For this review, take the finished solid that the model builds, in its own axes (mm). Coordinates: 2 decimals unless noted, no trailing zeros. Write each loop counter-clockwise with the first axis right and the second up, starting at its lowest first coordinate (ties: lowest second). Pieces come first, ordered by that corner, then holes. Notation, with made-up numbers: M 88,46 L 98,46 A16 cw 98,66 Z; hole C 33.5,72 d9. An arc over 180 degrees is marked long. One line per question, with ' | ' between items.
from build123d import *

# Parameters (mm, degrees)
F0_R     = 10.95
F1_DEPTH = 7
F2_R     = 1


with BuildPart() as f1:
    # F0 (on Top) → F1 (new body)
    with BuildSketch(Plane.XY):
        with BuildLine():
            ThreePointArc((-21.5356414958, -4.8959657474), (-23.8783924252, 3.2977389637), (-21.5356414958, 11.4914436749))
            ThreePointArc((-21.5356414958, 11.4914436749), (-22.6993144087, 13.1854483171), (-24.0705316121, 14.7163140059))
            ThreePointArc((-24.0705316121, 14.7163140059), (-24.150511625, 14.7916467191), (-24.2283924252, 14.8691476939))
            ThreePointArc((-24.2283924252, 14.8691476939), (-29.3261886183, 18.1493809552), (-35.2783924252, 19.2977389637))
            ThreePointArc((-35.2783924252, 19.2977389637), (-37.8102942344, 19.0961399344), (-40.2783924252, 18.4964231173))
            ThreePointArc((-40.2783924252, 18.4964231173), (-50.1108366069, -2.7021443349), (-28.305201053, -11.1027680443))
            ThreePointArc((-28.305201053, -11.1027680443), (-26.1407697818, -9.8363332314), (-24.200803492, -8.2472609682))
            ThreePointArc((-24.200803492, -8.2472609682), (-24.1495735944, -8.1967605248), (-24.0974438172, -8.14718953))
            ThreePointArc((-24.0974438172, -8.14718953), (-22.7109617539, -6.6047701285), (-21.5356414958, -4.8959657474))
        make_face()
        with Locations((-35.2783924252, 3.2977389637)):
            Circle(F0_R, mode=Mode.SUBTRACT)
        with BuildLine():
            ThreePointArc((-35.2783924252, 19.2977389637), (-13.6974768248, 21.3714318141), (6.7324567843, 14.1151288356))
            ThreePointArc((6.7324567843, 14.1151288356), (8.5674737327, 15.8243194809), (10.647013196, 17.2257956612))
            ThreePointArc((10.647013196, 17.2257956612), (-14.6417402019, 24.8328180176), (-40.2783924252, 18.4964231173))
            ThreePointArc((-40.2783924252, 18.4964231173), (-37.8102942344, 19.0961399344), (-35.2783924252, 19.2977389637))
        make_face()
        with BuildLine():
            ThreePointArc((-19.2986991166, 4.1035936434), (-8.3783924252, 14.2477389637), (2.5419142663, 4.1035936434))
            ThreePointArc((2.5419142663, 4.1035936434), (3.2081819329, 7.93443985), (4.7788566455, 11.4914436749))
            ThreePointArc((4.7788566455, 11.4914436749), (3.7989548826, 12.8874320009), (2.6716075748, 14.1673065724))
            ThreePointArc((2.6716075748, 14.1673065724), (-8.3783924252, 18.7977389637), (-19.4283924252, 14.1673065724))
            ThreePointArc((-19.4283924252, 14.1673065724), (-20.5557397329, 12.8874320009), (-21.5356414958, 11.4914436749))
            ThreePointArc((-21.5356414958, 11.4914436749), (-19.9649667832, 7.93443985), (-19.2986991166, 4.1035936434))
        make_face()
        with BuildLine():
            ThreePointArc((-19.2986991166, 2.4918842841), (-19.3283924252, 3.2977389637), (-19.2986991166, 4.1035936434))
            ThreePointArc((-19.2986991166, 4.1035936434), (-19.9649667832, 7.93443985), (-21.5356414958, 11.4914436749))
            ThreePointArc((-21.5356414958, 11.4914436749), (-23.8783924252, 3.2977389637), (-21.5356414958, -4.8959657474))
            ThreePointArc((-21.5356414958, -4.8959657474), (-19.9649667832, -1.3389619226), (-19.2986991166, 2.4918842841))
        make_face()
        with BuildLine():
            ThreePointArc((4.7788566455, -4.8959657474), (3.2081819329, -1.3389619226), (2.5419142663, 2.4918842841))
            ThreePointArc((2.5419142663, 2.4918842841), (-8.3783924252, -7.6522610363), (-19.2986991166, 2.4918842841))
            ThreePointArc((-19.2986991166, 2.4918842841), (-19.9649667832, -1.3389619226), (-21.5356414958, -4.8959657474))
            ThreePointArc((-21.5356414958, -4.8959657474), (-20.5557397329, -6.2919540734), (-19.4283924252, -7.571828645))
            ThreePointArc((-19.4283924252, -7.571828645), (-8.3783924252, -12.2022610363), (2.6716075748, -7.571828645))
            ThreePointArc((2.6716075748, -7.571828645), (3.7989548826, -6.2919540734), (4.7788566455, -4.8959657474))
        make_face()
        with BuildLine():
            ThreePointArc((2.5419142663, 4.1035936434), (2.5641817297, 3.7009397379), (2.5716075748, 3.2977389637))
            ThreePointArc((2.5716075748, 3.2977389637), (2.5641817297, 2.8945381895), (2.5419142663, 2.4918842841))
            ThreePointArc((2.5419142663, 2.4918842841), (3.2081819329, -1.3389619226), (4.7788566455, -4.8959657474))
            ThreePointArc((4.7788566455, -4.8959657474), (6.5244153739, -0.9632843526), (7.1216075748, 3.2977389637))
            ThreePointArc((7.1216075748, 3.2977389637), (6.5244153739, 7.5587622801), (4.7788566455, 11.4914436749))
            ThreePointArc((4.7788566455, 11.4914436749), (3.2081819329, 7.93443985), (2.5419142663, 4.1035936434))
        make_face()
        with BuildLine():
            ThreePointArc((6.7324567843, 14.1151288356), (5.6884305592, 12.8533429575), (4.7788566455, 11.4914436749))
            ThreePointArc((4.7788566455, 11.4914436749), (6.5244153739, 7.5587622801), (7.1216075748, 3.2977389637))
            ThreePointArc((7.1216075748, 3.2977389637), (6.5244153739, -0.9632843526), (4.7788566455, -4.8959657474))
            ThreePointArc((4.7788566455, -4.8959657474), (5.9425295584, -6.5899703896), (7.3137467617, -8.1208360785))
            ThreePointArc((7.3137467617, -8.1208360785), (7.3937267746, -8.1961687916), (7.4716075748, -8.2736697664))
            ThreePointArc((7.4716075748, -8.2736697664), (12.5694037679, -11.5539030277), (18.5216075748, -12.7022610363))
            ThreePointArc((18.5216075748, -12.7022610363), (21.0216075748, -12.5057416655), (23.4601952715, -11.9210110363))
            ThreePointArc((23.4601952715, -11.9210110363), (31.4641228471, -6.1092424026), (34.5216075748, 3.2977389637))
            ThreePointArc((34.5216075748, 3.2977389637), (26.584066565, 17.1178965255), (10.647013196, 17.2257956612))
            ThreePointArc((10.647013196, 17.2257956612), (8.5674737327, 15.8243194809), (6.7324567843, 14.1151288356))
        make_face()
        with Locations((18.5216075748, 3.2977389637)):
            Circle(F0_R, mode=Mode.SUBTRACT)
        with BuildLine():
            ThreePointArc((18.5216075748, -12.7022610363), (-3.3423713912, -15.2962408971), (-24.200803492, -8.2472609682))
            ThreePointArc((-24.200803492, -8.2472609682), (-26.1407697818, -9.8363332314), (-28.305201053, -11.1027680443))
            ThreePointArc((-28.305201053, -11.1027680443), (-2.5366521789, -18.7334401031), (23.4601952715, -11.9210110363))
            ThreePointArc((23.4601952715, -11.9210110363), (21.0216075748, -12.5057416655), (18.5216075748, -12.7022610363))
        make_face()
    extrude(amount=F1_DEPTH)

    # F2
    f2_edges = [f1.edges().sort_by_distance(p)[0] for p in [
        (7.571608, 3.297739, 7),
        (-19.298699, 2.491884, 7),
        (-46.228392, 3.297739, 7),
    ]]
    fillet(f2_edges, radius=F2_R)


solid = f1.part
1) We need section B-B on y = 20.5. State the section outline as (x, z) points, then the cut area to 3 significant figures.
Responses:
outline: M -36.28,0 L -30.92,0 L -30.92,7 L -36.28,7 Z; M -8.72,0 L 4.51,0 L 4.51,7 L -8.72,7 Z | area: 130 mm^2
2) We need section A-A on z = 3.75. State the section outline as (x, y) points, then the cut area to 3 significant figures.
Responses:
outline: M -40.28,18.5 A16 ccw long -28.31,-11.1 A50 ccw 23.46,-11.92 A16 ccw long 10.65,17.23 A50 ccw Z; hole C -35.28,3.3 d21.9; hole M -35.28,19.3 A16 cw -24.23,14.87 A4 ccw -24.07,14.72 A16 cw -21.54,11.49 A15.5 cw 4.78,11.49 A16 cw 6.73,14.12 A50 ccw Z; hole M -24.2,-8.25 A50 ccw 18.52,-12.7 A16 cw 7.47,-8.27 A4 ccw 7.31,-8.12 A16 cw 4.78,-4.9 A15.5 cw -21.54,-4.9 A16 cw -24.1,-8.15 A4 ccw Z; hole C -8.38,3.3 d21.9; hole C 18.52,3.3 d21.9 | area: 1,450 mm^2
3) To check wall thickness, follow line 1 along X through (y, z) = (11, 4.75); line 2 along Y through (x, z) = (-6, 6.25); line 3 along X through (y, z) = (-10.5, 6). State the ranges of each line that lie inside material, in increasing order. Write a range as [from, to].
Responses:
line 1: [-49.3, -43.06], [-27.5, -16.16], [-0.6, 10.74], [26.3, 32.55] | line 2: [-18.56, -14.95], [-12.02, -7.42], [14.02, 18.61], [19.8, 23.86] | line 3: [-43.38, -20.09], [-15.44, -1.32], [10.42, 26.62]
4) Insertion check: pin 1 Ø3 at (y, z) = (-6, 1) entering from -X; pin 2 Ø10 at (x, y) = (23.5, 12) entering from +Z; pin 3 Ø3 at (x, z) = (15.5, 1) entering from +Y; pin 4 Ø2 at (x, z) = (-6, 5.5) entering from -Y. Each pin has a flat end and moves straight along its axis. Give the tip position at first contact, or say it passes through.
Responses:
pin 1: x = -49.25 | pin 2: z = 7 | pin 3: y = 19.23 | pin 4: y = -18.63
5) The part is to be moulded in two halves that separate along X. For faces 1 (the flat face through (-18, 11, 7)), 2 (the cylindrical face through (-22.73, -6.63, 3.45)), say which applies: +X half, -X half, draft (parallel to the pull), parting line (faces both ways), or undercut.
Responses:
face 1: draft | face 2: undercut
6) We need section C-C on y = 0.5. State how many separate pieces and enclosed holes the cut face has, then the cut area to 3 significant figures.
Responses:
separate pieces: 4 | enclosed holes: 0 | area: 151 mm^2
